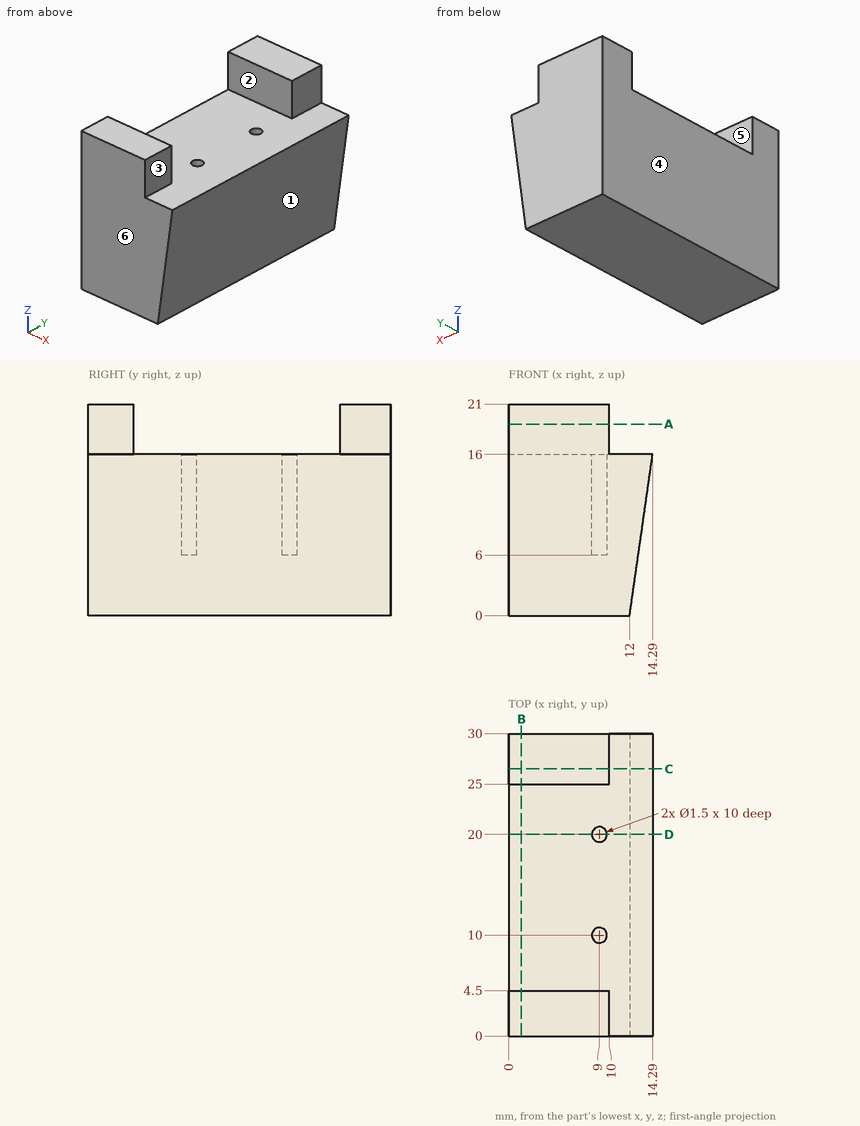
Geometry: see drawing. Coordinates: mm, zero at the bounding-box minimum. A direction names the side the tool comes from. Give positions to 0.01 mm unless a question says otherwise; leave off trailing zeros. Order: outer loops, then holes, each group sorted by start corner. A loop starts at its lowest first (then second) coordinate and runs counter-clockwise, first axis right, second up. Notation, with made-up numbers: (-7.5, -14) -> (19.5, -14) arc R31 cw to (19.5, 13) -> close; hole circle Ø11 at (-17.5, 60). An arc over 180 degrees is marked (long way). Write each question's results on one line, items separated by ' | '. Start each with the question number.
1) Draft query along Y for the marked faces 4, 5 and 6. Return one class per face: pulls with the +Y half, pulls with the -Y half, needs draft (parallel to the pull), parting line crosses it, or undercut.
2) Section B-B (x = 1.25). Return loops of the section in (y, z), then the cut area to 4 significant figures.
3) Section C-C (y = 26.5). Return loops of the section in (x, z).
4) Section D-D (y = 20). Return loops of the section in (x, z).
5) First-contact query: pin 1 (7 mm diameter, centred on x = 6.5, y = 19, fed in from +Z); pin 2 (5.5 mm diameter, centred on y = 28.5, z = 18.5, fed in from +X); pin 3 (2 mm diameter, centred on y = 2, z = 18.5, fed in from +X). Flat tips, straight axial feed; report the tip coordinate or a pass-through.
6) Line query: line 1 (Y direction, x = 9, z = 9.75); line 2 (Y direction, x = 9.75, z = 17.75); line 3 (Z direction, x = 11.25, y = 15.5). Output: solid intervals per line, ascending. Write a range as from..to.
7) Set-up query: the marked faces 1, 2 and 3. Return all of +Z, -Z, +X, -X, +Y, -Y with unobstructed straight access to the full face (end or side cutting, diameter ignored); none if empty.
8) Section A-A (z = 19). Return loops of the section in (x, y).
Calculated:
1) face 4: needs draft | face 5: undercut | face 6: pulls with the -Y half
2) outline: (0, 0) -> (30, 0) -> (30, 21) -> (25, 21) -> (25, 16) -> (4.5, 16) -> (4.5, 21) -> (0, 21) -> close | area: 527.5 mm2
3) outline: (0, 0) -> (12, 0) -> (14.29, 16) -> (10, 16) -> (10, 21) -> (0, 21) -> close
4) outline: (0, 0) -> (12, 0) -> (14.29, 16) -> (9.75, 16) -> (9.75, 6) -> (8.25, 6) -> (8.25, 16) -> (0, 16) -> close
5) pin 1: z = 16 | pin 2: x = 14.29 | pin 3: x = 10
6) line 1: 0..9.25, 10.75..19.25, 20.75..30 | line 2: 0..4.5, 25..30 | line 3: 0..16
7) face 1: -Z, +X, +Y, -Y | face 2: +Z, +X, -X | face 3: +Z, +X, +Y, -Y
8) outline: (0, 0) -> (10, 0) -> (10, 4.5) -> (0, 4.5) -> close; (0, 25) -> (10, 25) -> (10, 30) -> (0, 30) -> close
